from build123d import *

# Parameters (mm, degrees)
F0_R     = 6
F1_DEPTH = 10
F2_R     = 10
F3_DEPTH = 8


with BuildPart() as f1:
    # F0 (on Top) → F1 (new body)
    with BuildSketch(Plane.XY):
        with BuildLine():
            ThreePointArc((0.720724, -17.985565), (12.980236, -12.470505), (18, 0))
            ThreePointArc((18, 0), (12.980236, 12.470505), (0.720724, 17.985565))
            ThreePointArc((0.720724, 17.985565), (-18, 0), (0.720724, -17.985565))
        make_face()
        Circle(F0_R, mode=Mode.SUBTRACT)
        with BuildLine():
            ThreePointArc((0.720724, -17.985565), (-18, 0), (0.720724, 17.985565))
            ThreePointArc((0.720724, 17.985565), (-19.637945, 23.224109), (-36.043982, 36.367918))
            ThreePointArc((-36.043982, 36.367918), (-33.041104, 31.032896), (-32, 25))
            ThreePointArc((-32, 25), (-49.804119, 7.001066), (-67.995737, 24.608261))
            Line((-67.995737, 24.608261), (-67.995737, -24.608261))
            ThreePointArc((-67.995737, -24.608261), (-49.804119, -7.001066), (-32, -25))
            ThreePointArc((-32, -25), (-33.041104, -31.032896), (-36.043982, -36.367918))
            ThreePointArc((-36.043982, -36.367918), (-19.637945, -23.224109), (0.720724, -17.985565))
        make_face()
        with BuildLine():
            ThreePointArc((-32, 25), (-33.041104, 31.032896), (-36.043982, 36.367918))
            ThreePointArc((-36.043982, 36.367918), (-55.847988, 42.023544), (-67.995737, 25.391739))
            Line((-67.995737, 25.391739), (-67.995737, 24.608261))
            ThreePointArc((-67.995737, 24.608261), (-49.804119, 7.001066), (-32, 25))
        make_face()
        with Locations((-50, 25)):
            Circle(F0_R, mode=Mode.SUBTRACT)
        with BuildLine():
            ThreePointArc((-67.995737, -25.391739), (-55.847988, -42.023544), (-36.043982, -36.367918))
            ThreePointArc((-36.043982, -36.367918), (-33.041104, -31.032896), (-32, -25))
            ThreePointArc((-32, -25), (-49.804119, -7.001066), (-67.995737, -24.608261))
            Line((-67.995737, -24.608261), (-67.995737, -25.391739))
        make_face()
        with Locations((-50, -25)):
            Circle(F0_R, mode=Mode.SUBTRACT)
        with BuildLine():
            Line((-67.995737, 24.608261), (-67.995737, 25.391739))
            ThreePointArc((-67.995737, 25.391739), (-68, 25), (-67.995737, 24.608261))
        make_face()
        with BuildLine():
            ThreePointArc((-67.995737, -24.608261), (-68, -25), (-67.995737, -25.391739))
            Line((-67.995737, -25.391739), (-67.995737, -24.608261))
        make_face()
    extrude(amount=F1_DEPTH)

    # F2 (on Front) → F3 (join, symmetric)
    with BuildSketch(Plane.XZ):
        with BuildLine():
            ThreePointArc((-16.430688, 10), (-58.939191, 17.449895), (-96.380751, 38.911565))
            ThreePointArc((-96.380751, 38.911565), (-131.140781, 29.481496), (-110.451962, 0))
            Line((-110.451962, 0), (-16.430688, 0))
            Line((-16.430688, 0), (-16.430688, 10))
        make_face()
        with Locations((-110.451962, 22)):
            Circle(F2_R, mode=Mode.SUBTRACT)
    extrude(amount=F3_DEPTH, both=True)


solid = f1.part
Part model, mm, in its own coordinate system. A direction names the side the tool comes from. Coordinates: 2 decimals unless noted, no trailing zeros. Write each loop counter-clockwise with the first axis right and the second up, starting at its lowest first coordinate (ties: lowest second). Pieces come first, ordered by that corner, then holes. Notation, with made-up numbers: (44, -12) - (62, -12) arc R9 cw to (62, -6) - close; hole circle Ø6 at (-25, -25). An arc over 180 degrees is marked (long way). Put each result on its own line as item: value.
1. 3-axis set-ups, long thin cutter, end or side, ignore diameter. For faces 4 (the cylindrical face through (-19.903, -23.358, 4.93)), 5 (the flat face through (-67.996, -16, 5)), 6 (the flat face through (-67.996, 16, 5)): which of +Z, -Z, +X, -X, +Y, -Y reach the whole face in a straight line?
Final values:
face 4: +Z, -Z, +X, -Y
face 5: +Z, -Z, -X, -Y
face 6: +Z, -Z, -X, +Y
2. Band-saw the part on B-B (x = -117.5). Write the cut outline in (y, z).
Final values:
outline: (-8, 1.16) - (8, 1.16) - (8, 14.91) - (-8, 14.91) - close; (-8, 29.09) - (8, 29.09) - (8, 42.84) - (-8, 42.84) - close
3. Probe line 1 along Y through (x, z) = (-50, 7.25); line 2 along Z through (x, y) = (-54.5, 9); line 3 along Y through (x, z) = (-81, 14). List the from-to ranges inside material, lowest first. Write a range as [from, to].
Final values:
line 1: y = [-43, -31], [-19, 19], [31, 43]
line 2: z = [0, 10]
line 3: y = [-8, 8]
4. Band-saw the part on C-C (x = -50). Write the cut outline in (y, z).
Final values:
outline: (-43, 0) - (-31, 0) - (-31, 10) - (-43, 10) - close; (-19, 0) - (19, 0) - (19, 10) - (8, 10) - (8, 14.59) - (-8, 14.59) - (-8, 10) - (-19, 10) - close; (31, 0) - (43, 0) - (43, 10) - (31, 10) - close
5. Band-saw the part on D-D (y = 32.5). Write the cut outline in (x, z).
Final values:
outline: (-66.36, 0) - (-32.54, 0) - (-32.54, 10) - (-66.36, 10) - close
6. Band-saw the part on A-A (z = 26.5). Write the cut outline in (x, y), then the cut area to 3 significant figures.
Final values:
outline: (-131.99, -8) - (-119.38, -8) - (-119.38, 8) - (-131.99, 8) - close; (-101.52, -8) - (-78.5, -8) - (-78.5, 8) - (-101.52, 8) - close
area: 570 mm²
7. Flat gauge pins, fed straight in: pin 1 Ø10 at (y, z) = (2, 30) entering from -X; pin 2 Ø5 at (y, z) = (-17.5, 5) entering from -X; pin 3 Ø3 at (y, z) = (-3.5, 28.5) entering from -X; pin 4 Ø15.5 at (x, y) = (-50, -25) entering from -Z. Where does each tip first touch, or does it go through?
Final values:
pin 1: stops at x = -132.25
pin 2: stops at x = -68
pin 3: stops at x = -131.88
pin 4: stops at z = 0
8. Two-plate mould, pull along X, no slides. Class faces 1 (the cylindrical face through (-56, -25, 5)), 2 (the flat face through (-47, -1, 0)), 3 (the cylindrical face through (-19.37, 23.09, 4.93)): +X half, -X half, draft (parallel to the pull), parting line (faces both ways), or undercut.
Final values:
face 1: undercut
face 2: draft
face 3: +X half
